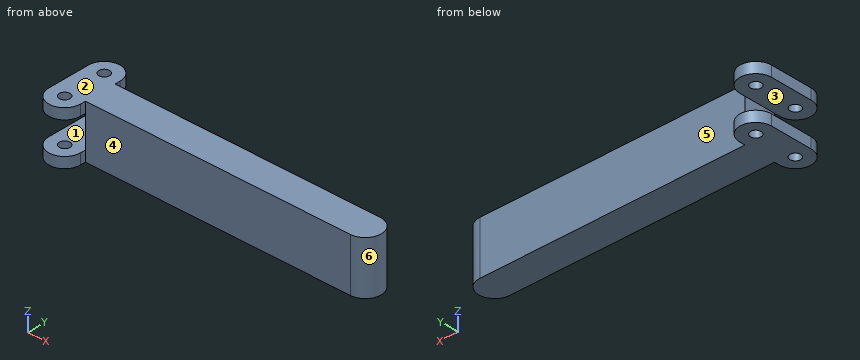
from build123d import *

# Parameters (mm, degrees)
SKETCH1_R           = 3.175
BOSS_EXTRUDE1_DEPTH = 31.75
SKETCH2_W           = 19.05
SKETCH2_H           = 25.4
SKETCH2_H_2         = 9.525
CUT_EXTRUDE1_DEPTH  = 19.05


with BuildPart() as part:
    # Sketch1 → Boss-Extrude1 (new body)
    with BuildSketch(Plane.XY):
        with BuildLine():
            Line((-9.525, 25.4), (-9.525, 0))
            ThreePointArc((-9.525, 0), (0, -9.525), (9.525, 0))
            Line((9.525, 0), (9.525, 3.175))
            Line((9.525, 3.175), (168.275, 3.175))
            ThreePointArc((168.275, 3.175), (177.8, 12.7), (168.275, 22.225))
            Line((168.275, 22.225), (9.525, 22.225))
            Line((9.525, 22.225), (9.525, 25.4))
            ThreePointArc((9.525, 25.4), (0, 34.925), (-9.525, 25.4))
        make_face()
        Circle(SKETCH1_R, mode=Mode.SUBTRACT)
        with Locations((0, 25.4)):
            Circle(SKETCH1_R, mode=Mode.SUBTRACT)
    extrude(amount=BOSS_EXTRUDE1_DEPTH)

    # Sketch2 → Cut-Extrude1 (cut)
    with BuildSketch(Plane.ZY.offset(9.525)):
        with Locations((15.875, 12.7)):
            Rectangle(SKETCH2_W, SKETCH2_H)
        with Locations((15.875, 30.1625)):
            Rectangle(SKETCH2_W, SKETCH2_H_2)
        with Locations((15.875, -4.7625)):
            Rectangle(SKETCH2_W, SKETCH2_H_2)
    extrude(amount=-CUT_EXTRUDE1_DEPTH, mode=Mode.SUBTRACT)


solid = part.part
Design review of the part built by this model. Coordinates are the model's own, in mm. Face numbers are marked on the shaded views. A direction names the side the tool comes from. Round coordinates to 2 decimals unless told otherwise and drop trailing zeros. Write each loop counter-clockwise with the first axis right and the second up, starting at its lowest first coordinate (ties: lowest second). Pieces come first, ordered by that corner, then holes. Notation, with made-up numbers: (-5.5, -22.5) -> (25.5, -22.5) arc R21 ccw to (25.5, 4.5) -> close; hole circle Ø5 at (-40, 61). An arc over 180 degrees is marked (long way). One line per item, written item: value. Start each with the question number.
Q1. Tool access review of the marked faces 5 and 6: name each direction out of +Z, -Z, +X, -X, +Y, -Y from which nothing blocks a thin tool from reaching the whole face with its end or side.
Q2. Add section B-B (y = 12.7). Give the boundary of the cut face in (x, z) (3 decimals).
Q3. Add section A-A (x = 0). Give the boundary of the cut face in (y, z) (3 decimals).
Q4. To check wall thickness, follow probe 1 along Y at (x, z) = (0, 29) (3 decimals); probe 2 along X at (y, z) = (25, 3) (3 decimals); probe 3 along Z at (x, y) = (5, 20). State the ranges of each line that lie inside material, in increasing order.
Q5. The part is to be moulded in two halves that separate along Z. For the marked faces 1, 2, 3 and 4, say which applies: pulls with the +Z half, pulls with the -Z half, needs draft (parallel to the pull), parting line crosses it, or undercut.
Q6. Add section C-C (z = 4). Give the boundary of the cut face in (x, y) (3 decimals), then the cut area to 3 significant figures.
Q7. Add section D-D (y = -5). Give the boundary of the cut face in (x, z), then the cut area to 3 significant figures.
Q8. Insertion check: P1, Ø16, axis at x = 82.5, z = 11.5, coming from the +Y side (3 decimals); P2, Ø12, axis at x = 106.5, z = 28, coming from the -Y side (3 decimals); P3, Ø2.5, axis at y = 24, z = 2, coming from the +X side (3 decimals). Each pin has a flat end and moves straight along its axis. Give the tip position at first contact, or say it passes through.
Response:
1. face 5: +Z, -Z, +X, +Y
1. face 6: +Z, -Z, +X
2. outline: (-9.525, 0) -> (177.8, 0) -> (177.8, 31.75) -> (-9.525, 31.75) -> (-9.525, 25.4) -> (9.525, 25.4) -> (9.525, 6.35) -> (-9.525, 6.35) -> close
3. outline: (-9.525, 0) -> (-3.175, 0) -> (-3.175, 6.35) -> (-9.525, 6.35) -> close; (-9.525, 25.4) -> (-3.175, 25.4) -> (-3.175, 31.75) -> (-9.525, 31.75) -> close; (3.175, 0) -> (22.225, 0) -> (22.225, 6.35) -> (3.175, 6.35) -> close; (3.175, 25.4) -> (22.225, 25.4) -> (22.225, 31.75) -> (3.175, 31.75) -> close; (28.575, 0) -> (34.925, 0) -> (34.925, 6.35) -> (28.575, 6.35) -> close; (28.575, 25.4) -> (34.925, 25.4) -> (34.925, 31.75) -> (28.575, 31.75) -> close
4. probe 1: y = -9.525 to -3.175, 3.175 to 22.225, 28.575 to 34.925
4. probe 2: x = -9.525 to -3.15, 3.15 to 9.525
4. probe 3: z = 0 to 6.35, 25.4 to 31.75
5. face 1: undercut
5. face 2: pulls with the +Z half
5. face 3: undercut
5. face 4: needs draft
6. outline: (-9.525, 0) arc R9.525 ccw to (9.525, 0) -> (9.525, 3.175) -> (168.275, 3.175) arc R9.525 ccw to (168.275, 22.225) -> (9.525, 22.225) -> (9.525, 25.4) arc R9.525 ccw to (-9.525, 25.4) -> close; hole circle Ø6.35 at (0, 0); hole circle Ø6.35 at (0, 25.4)
6. area: 3,870 mm^2
7. outline: (-8.11, 0) -> (8.11, 0) -> (8.11, 6.35) -> (-8.11, 6.35) -> close; (-8.11, 25.4) -> (8.11, 25.4) -> (8.11, 31.75) -> (-8.11, 31.75) -> close
7. area: 206 mm^2
8. P1: stops at y = 22.225
8. P2: stops at y = 3.175
8. P3: stops at x = 9.525
